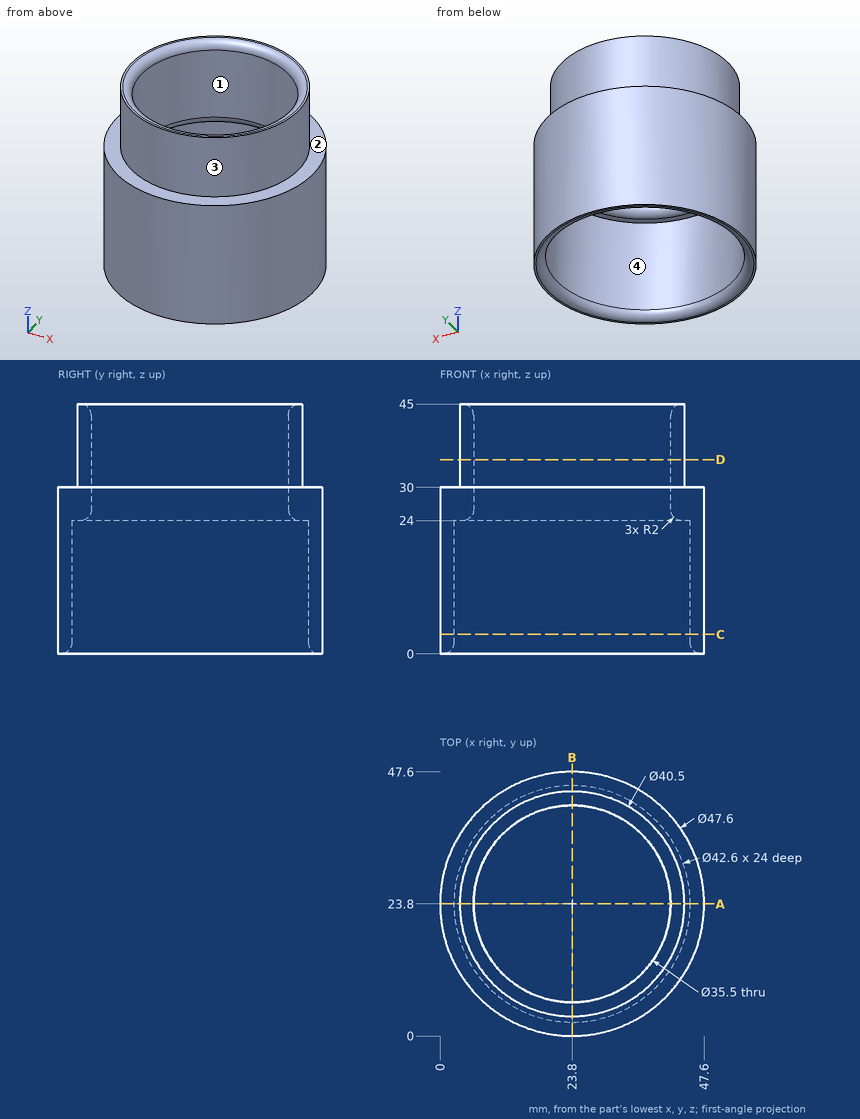
Can you work these out from the drawing? Everything is in mm from the part's minimum corner. Round coordinates to 2 decimals unless told otherwise and drop trailing zeros. Write each loop counter-clockwise with the first axis right and the second up, starting at its lowest first coordinate (ties: lowest second). Pieces come first, ordered by that corner, then holes. Notation, with made-up numbers: M 18,23.5 L 64,23.5 A28 cw 64,59.5 Z; hole C -22.5,83.25 d3. An arc over 180 degrees is marked long. Use a Markdown table: item, result.
Item 1: I want a section at A-A (y = 23.8). List the corners of the cut face in (x, z) for me.
Found:
| item | result |
|---|---|
| outline | M 0,0 L 0.5,0 A2 ccw 2.5,2 L 2.5,24 L 4.05,24 A2 ccw 6.05,26 L 6.05,43 A2 ccw 4.05,45 L 3.55,45 L 3.55,30 L 0,30 Z; M 41.55,26 A2 ccw 43.55,24 L 45.1,24 L 45.1,2 A2 ccw 47.1,0 L 47.6,0 L 47.6,30 L 44.05,30 L 44.05,45 L 43.55,45 A2 ccw 41.55,43 Z |
Item 2: For pin 1 Ø3 at (y, z) = (35, 4.5) entering from -X; pin 2 Ø4 at (x, y) = (36, 40.5) entering from -Z; pin 3 Ø8 at (y, z) = (16, 8) entering from +X, each with a flat end and sliding along its axis, tell me the tip position at first contact or that it passes through.
Found:
| item | result |
|---|---|
| pin 1 | stops at x = 2.07 |
| pin 2 | stops at z = 0.1 |
| pin 3 | stops at x = 47.29 |
Item 3: I want a section at D-D (z = 35). List the corners of the cut face in (x, y) for me, and give its area (3 significant figures).
Found:
| item | result |
|---|---|
| outline | C 23.8,23.8 d40.5; hole C 23.8,23.8 d35.5 |
| area | 298 mm2 |
Item 4: We'd pull the mould along X, two halves only. Please class the marked faces 1, 2, 3 and 4: released by +X, released by -X, zero draft, split by the parting line, or undercut.
Found:
| item | result |
|---|---|
| face 1 | undercut |
| face 2 | zero draft |
| face 3 | split by the parting line |
| face 4 | undercut |
Item 5: I want a section at C-C (z = 3.5). List the corners of the cut face in (x, y) for me.
Found:
| item | result |
|---|---|
| outline | C 23.8,23.8 d47.6; hole C 23.8,23.8 d42.6 |
Item 6: If I drill on line 1 along Y through (x, z) = (23, 9.5); line 2 along X through (y, z) = (13, 41.5); line 3 along X through (y, z) = (37, 24.5), over which ranges is the centre line in solid material (lowest first)? Write a range as [from, to].
Found:
| item | result |
|---|---|
| line 1 | y = [0.01, 2.52], [45.08, 47.59] |
| line 2 | x = [6.67, 9.71], [37.89, 40.93] |
| line 3 | x = [4, 10.94], [36.66, 43.6] |
